Could you check a few things on this model? Use its own coordinates, in mm. Face numbers are marked on the shaded views. A direction names the side the tool comes from. Coordinates: 2 decimals unless noted, no trailing zeros. Write each loop counter-clockwise with the first axis right and the second up, starting at its lowest first coordinate (ties: lowest second). Pieces come first, ordered by that corner, then holes.
Item 1: I want a section at C-C on x = 8. Please give me the cut outline in (y, z), then the cut area to 3 significant figures.
Item 2: For P1, Ø1.5, axis at x = 8.5, y = -8.5, coming from the -Z side; P2, Ø13.5, axis at x = 8, y = 0, coming from the +Z side; P3, Ø6.5, axis at x = -8, y = 0, coming from the +Z side, each with a flat end and sliding along its axis, tell me the tip position at first contact or that it passes through.
Item 3: Which directions (+Z, -Z, +X, -X, +Y, -Y) give clear straight access to the entire face, cutting with the end or side of a thin tool? Please do the marked faces 1 and 2.
Item 4: Thinking about a two-plate mould opening in X: for the marked faces 3, 4 and 5, which applies, +X half, -X half, draft (parallel to the pull), parting line (faces both ways), or undercut?
Item 5: I want a section at A-A on x = 0. Please give me the cut outline in (y, z).
Item 6: I want a section at D-D on y = 0. Please give me the cut outline in (x, z), then the cut area to 3 significant figures.
Item 7: If I drill on probe 1 along Y at (x, z) = (-13, 20); probe 2 along Y at (x, z) = (-8, 4.75); probe 3 along Z at (x, y) = (0, -22), over which ranges is the centre line in solid material (lowest first)?
Item 8: I want a section at B-B on z = 15.5. Please give me the cut outline in (x, y), then the cut area to 3 significant figures.
from build123d import *

# Parameters (mm, degrees)
SKETCH1_W           = 34.6
SKETCH1_H           = 50
SKETCH1_R           = 4.2
BOSS_EXTRUDE1_DEPTH = 30
SKETCH2_W           = 20
SKETCH2_H           = 30
CUT_EXTRUDE1_DEPTH  = 35.6
SKETCH3_R           = 3.15
CUT_EXTRUDE2_DEPTH  = 51


with BuildPart() as part:
    # Sketch1 → Boss-Extrude1 (new body)
    with BuildSketch(Plane.XY):
        Rectangle(SKETCH1_W, SKETCH1_H)
        with Locations((-8, 0)):
            Circle(SKETCH1_R, mode=Mode.SUBTRACT)
        with Locations((8, 0)):
            Circle(SKETCH1_R, mode=Mode.SUBTRACT)
    extrude(amount=BOSS_EXTRUDE1_DEPTH)

    # Sketch2 → Cut-Extrude1 (cut, through all)
    with BuildSketch(Plane.ZY.offset(17.3)):
        with Locations((20, 0)):
            Rectangle(SKETCH2_W, SKETCH2_H)
    extrude(amount=-CUT_EXTRUDE1_DEPTH, mode=Mode.SUBTRACT)

    # Sketch3 → Cut-Extrude2 (cut, through all)
    with BuildSketch(Plane(origin=(0, 25, 0), x_dir=(1, 0, 0), z_dir=(0, 1, 0))):
        with Locations((0, -20)):
            Circle(SKETCH3_R)
    extrude(amount=-CUT_EXTRUDE2_DEPTH, mode=Mode.SUBTRACT)


solid = part.part
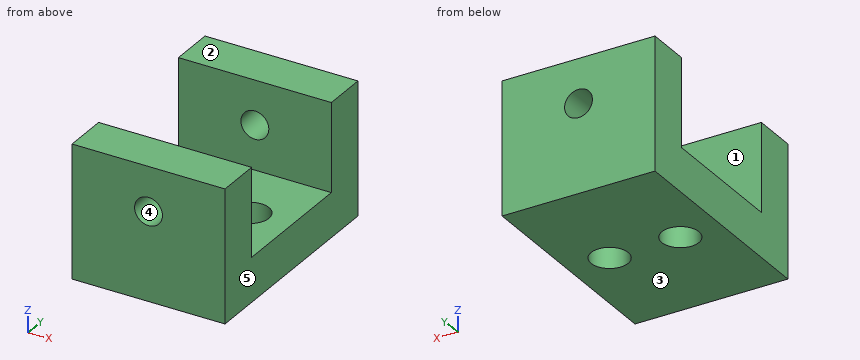
Response values:
1. outline: (-25, 0) - (-4.2, 0) - (-4.2, 10) - (-15, 10) - (-15, 30) - (-25, 30) - close; (4.2, 0) - (25, 0) - (25, 30) - (15, 30) - (15, 10) - (4.2, 10) - close
1. area: 816 mm2
2. P1: stops at z = 0
2. P2: stops at z = 10
2. P3: passes through
3. face 1: +Z, +X, -X
3. face 2: +Z, +X, -X, +Y, -Y
4. face 3: draft
4. face 4: undercut
4. face 5: +X half
5. outline: (-25, 0) - (25, 0) - (25, 16.85) - (15, 16.85) - (15, 10) - (-15, 10) - (-15, 16.85) - (-25, 16.85) - close; (-25, 23.15) - (-15, 23.15) - (-15, 30) - (-25, 30) - close; (15, 23.15) - (25, 23.15) - (25, 30) - (15, 30) - close
6. outline: (-17.3, 0) - (-12.2, 0) - (-12.2, 10) - (-17.3, 10) - close; (-3.8, 0) - (3.8, 0) - (3.8, 10) - (-3.8, 10) - close; (12.2, 0) - (17.3, 0) - (17.3, 10) - (12.2, 10) - close
6. area: 178 mm2
7. probe 1: y = -25 to -15, 15 to 25
7. probe 2: y = -25 to -4.2, 4.2 to 25
7. probe 3: z = 0 to 16.85, 23.15 to 30
8. outline: (-17.3, -25) - (17.3, -25) - (17.3, -15) - (-17.3, -15) - close; (-17.3, 15) - (17.3, 15) - (17.3, 25) - (-17.3, 25) - close
8. area: 692 mm2
